Verification items for this drawing (mm, ordinates from the low corner). A direction names the side the tool comes from. Round coordinates to 2 decimals unless told otherwise and drop trailing zeros. Write each loop counter-clockwise with the first axis right and the second up, starting at its lowest first coordinate (ties: lowest second). Pieces come first, ordered by that corner, then holes. Notation, with made-up numbers: (-18, 25.25) -> (11, 25.25) arc R13 ccw to (11, 46.25) -> close; hole circle Ø8 at (35, -22.5). An arc over 180 degrees is marked (long way). Use one line per item in the form item = value. Start each with the question number.
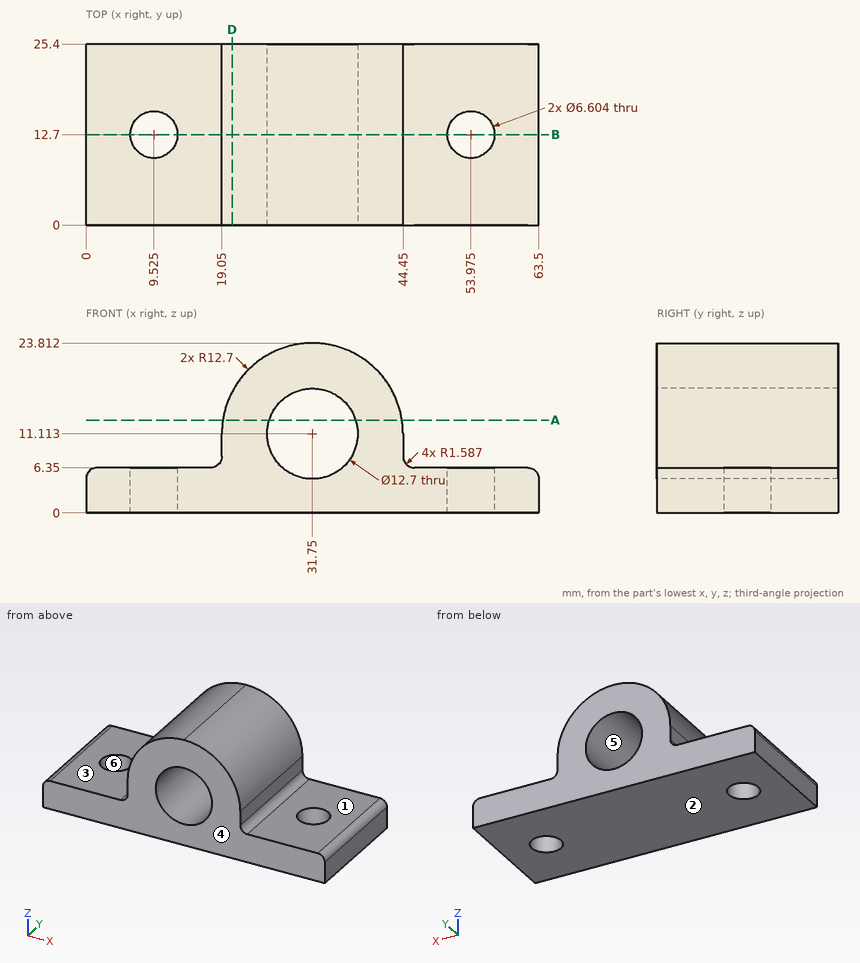
1. Mould release check, pull along Y, two halves, no side actions. Record for the marked faces 4, 5 and 6: +Y half, -Y half, draft (parallel to the pull), parting line (faces both ways), or undercut.
2. Scan lines: probe 1 along Z at (x, y) = (31.75, 12.5); probe 2 along X at (y, z) = (11.75, 3.25); probe 3 along Z at (x, y) = (4, 6.75). Record each from-to range of solid material in increasing order.
3. Sectioned sample at A-A (z = 13). Enter the section's corners in (x, y).
4. Sectioned sample at D-D (x = 20.5). Enter the section's corners in (y, z) (1 decimal), and give its area (3 significant figures).
5. Depth check by flat-ended pin: pin 1 (8 mm diameter, centred on x = 52, y = 15.5, fed in from -Z); pin 2 (3.5 mm diameter, centred on y = 13, z = 10.5, fed in from -X); pin 3 (8 mm diameter, centred on x = 5.5, y = 11, fed in from +Z); pin 4 (4 mm diameter, centred on x = 53.975, y = 12.7, fed in from +Z). Enter the tip coordinate at first touch or a pass-through.
6. Tool access check on the marked faces 1, 2 and 3. Record the directions out of +Z, -Z, +X, -X, +Y, -Y that give a thin tool (end or side, any length) a straight path to the whole face; none if there is none.
7. Sectioned sample at B-B (y = 12.7). Give the number of separate pieces and of enclosed holes in the cut face, and give its area (3 significant figures).
Returned:
q1.face_4 = -Y half
q1.face_5 = draft
q1.face_6 = undercut
q2.probe_1 = 0 to 4.76, 17.46 to 23.81
q2.probe_2 = 0 to 6.36, 12.69 to 50.81, 57.14 to 63.5
q2.probe_3 = 0 to 6.35
q3.outline = (19.19, 0) -> (25.69, 0) -> (25.69, 25.4) -> (19.19, 25.4) -> close; (37.81, 0) -> (44.31, 0) -> (44.31, 25.4) -> (37.81, 25.4) -> close
q4.outline = (0, 0) -> (25.4, 0) -> (25.4, 17) -> (0, 17) -> close
q4.area = 432 mm^2
q5.pin_1 = 0
q5.pin_2 = 19.05
q5.pin_3 = 6.35
q5.pin_4 = through
q6.face_1 = +Z, +X, +Y, -Y
q6.face_2 = -Z, +X, -X, +Y, -Y
q6.face_3 = +Z, -X, +Y, -Y
q7.separate_pieces = 3
q7.enclosed_holes = 1
q7.area = 567 mm^2
